Here's how the part is built. I have some questions about the finished solid (model axes, mm). Face numbers are marked on the shaded views. A direction names the side the tool comes from. Round coordinates to 2 decimals unless told otherwise and drop trailing zeros. Loops run counter-clockwise (first coordinate to the right, second up) from the corner with the lowest first, then second, coordinate; pieces in that order, holes last. Notation, with made-up numbers: (0, 44) -> (28, 44) arc R27 cw to (28, 62) -> close; hole circle Ø3 at (30, -9.75). An arc over 180 degrees is marked (long way). One line per item, written item: value. Start each with the question number.
Autodesk Inventor part; units mm, degrees
ref_plane "YZ Plane" through (0, 0, 0) normal (1, 0, 0) x (0, 1, 0)
ref_plane "XZ Plane" through (0, 0, 0) normal (0, 1, 0) x (-1, 0, 0)
ref_plane "XY Plane" through (0, 0, 0) normal (0, 0, 1) x (1, 0, 0)
sketch "스케치1" plane through (0, 0, 0) normal (0, 1, 0) x (-1, 0, 0)
  line L0 (-27.5, 10) -> (27.5, 10)
  line L1 (27.5, 10) -> (27.5, -10)
  line L2 (27.5, -10) -> (-27.5, -10)
  line L3 (-27.5, -10) -> (-27.5, 10)
  line L4 (-27.5, 10) -> (27.5, -10) construction
  line L5 (27.5, 10) -> (-27.5, -10) construction
  line L6 (-27.5, 10) -> (-24.5, 10)
  line L7 (-24.5, 10) -> (-24.5, -10)
  line L8 (-24.5, -10) -> (-27.5, -10)
  line L9 (-27.5, -10) -> (-27.5, 10)
  circle A0 centre (20, 0) radius 1.25
  circle A1 centre (-20, 0) radius 1.25
  point P0 (0, 0)
  dimension "d0" = 55
  dimension "d1" = 20
  dimension "d5" = 3
  dimension "d14" = 2.5
  dimension "d15" = 2.5
  dimension "d17" = 47.5
  dimension "d18" = 7.5
extrude "돌출1" add sketch "스케치1" along normal blind 3
extrude "돌출2" add sketch "스케치1" against normal blind 17.2 contours L0 L7 L2 L3
sketch "스케치2" plane through (24.5, -17.2, -10) normal (-1, 0, 0) x (0, 0, 1)
  line L0 (20, 17.2) -> (20, 0)
  line L1 (0, 17.2) -> (20, 17.2)
  line L2 (0, 17.2) -> (0, 0)
  line L3 (20, 0) -> (0, 0)
  line L4 (20, 17.2) -> (20, 0)
  circle A0 centre (10, 5) radius 2.5
  circle A1 centre (10, 5) radius 3.5
  point P0 (10, 17.2)
  point P1 (10, 0)
  dimension "d8" = 5
  dimension "d9" = 5
  dimension "d10" = 7
chamfer "모따기1" distance 2 angle 45 1 edges at (24.5, 0, 0)
extrude "돌출3" cut sketch "스케치2" against normal blind 3 contours A0
sketch "스케치5" plane through (27.5, 3, 10) normal (1, 0, 0) x (0, 0, -1)
  line L0 (0, -20.2) -> (0, 0)
  line L1 (20, -20.2) -> (0, -20.2)
  line L2 (7, -10.7) -> (13, -10.7)
  line L3 (20, -20.2) -> (20, 0)
  line L4 (10, -3) -> (10, -10.7) construction
  line L5 (7, -10.7) -> (7, -6.7)
  line L6 (13, -10.7) -> (13, -6.7)
  line L7 (7, -6.7) -> (13, -6.7)
  line L8 (20, -6.7) -> (20.03, -6.7)
  point P0 (7, -8.7)
  dimension "d33" = 3
extrude "돌출5" add sketch "스케치5" along normal blind 2
properties part number "base"
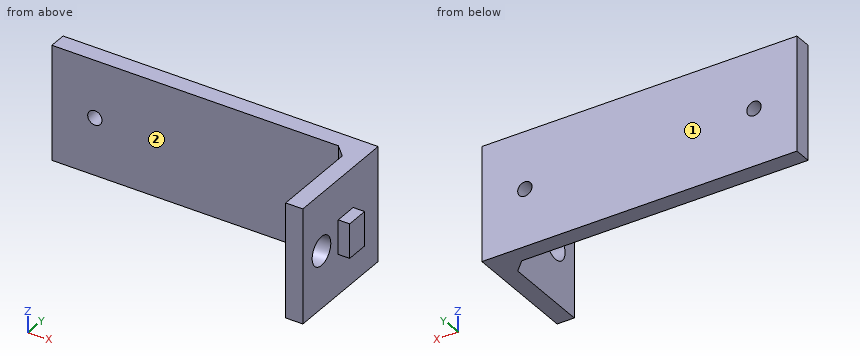
Q1. I want a section at A-A on y = -12.2. Please give me the cut outline in (x, z).
Q2. I want a section at D-D on z = 4.5. Please give me the cut outline in (x, y).
Q3. Which directions (+Z, -Z, +X, -X, +Y, -Y) give clear straight access to the entire face, cutting with the end or side of a thin tool? Please do the marked faces 1 and 2.
Q4. I want a section at C-C on z = 0. Please give me the cut outline in (x, y).
Q5. Will these pins go through, and if not, where does the flat tip stop? P1, Ø2, axis at x = 29, z = 1, coming from the +Y side; P2, Ø3, axis at x = 20, z = 0, coming from the -Y side; P3, Ø4.5, axis at y = -9, z = 4.5, coming from the -X side.
Q6. If I drill on line 1 along Z through (x, y) = (20, 1.7); line 2 along X through (y, z) = (-5, 1.5); line 3 along Y through (x, z) = (-6.5, -9), over which ranges is the centre line in solid material (lowest first)?
Q7. I want a section at B-B on x = -20. Please give me the cut outline in (y, z).
Answers below:
1. outline: (24.5, -10) -> (27.5, -10) -> (27.5, -2.5) -> (24.5, -2.5) -> close; (24.5, 2.5) -> (27.5, 2.5) -> (27.5, 10) -> (24.5, 10) -> close
2. outline: (-27.5, 0) -> (22.5, 0) -> (24.5, -2) -> (24.5, -17.2) -> (27.5, -17.2) -> (27.5, 3) -> (-27.5, 3) -> close
3. face 1: +Z, -Z, +X, -X, +Y
3. face 2: +Z, -Z, -X, -Y
4. outline: (-27.5, 0) -> (-21.25, 0) -> (-21.25, 3) -> (-27.5, 3) -> close; (-18.75, 0) -> (18.75, 0) -> (18.75, 3) -> (-18.75, 3) -> close; (21.25, 0) -> (22.5, 0) -> (24.5, -2) -> (24.5, -9.7) -> (27.5, -9.7) -> (27.5, -7.7) -> (29.5, -7.7) -> (29.5, -3.7) -> (27.5, -3.7) -> (27.5, 3) -> (21.25, 3) -> close; (24.5, -17.2) -> (27.5, -17.2) -> (27.5, -14.7) -> (24.5, -14.7) -> close
5. P1: stops at y = -3.7
5. P2: stops at y = 0
5. P3: stops at x = 24.5
6. line 1: z = -10 to -1.25, 1.25 to 10
6. line 2: x = 24.5 to 29.5
6. line 3: y = 0 to 3
7. outline: (0, -10) -> (3, -10) -> (3, -1.25) -> (0, -1.25) -> close; (0, 1.25) -> (3, 1.25) -> (3, 10) -> (0, 10) -> close
